Autodesk Inventor part; units mm, degrees
ref_plane "YZ Plane" through (0, 0, 0) normal (1, 0, 0) x (0, 1, 0)
ref_plane "XZ Plane" through (0, 0, 0) normal (0, 1, 0) x (-1, 0, 0)
ref_plane "XY Plane" through (0, 0, 0) normal (0, 0, 1) x (1, 0, 0)
sketch "Sketch1" plane through (0, 0, 0) normal (0, 0, 1) x (1, 0, 0)
  line L0 (0, 0) -> (30, 0)
  line L1 (30, 0) -> (30, 10)
  line L2 (30, 10) -> (0, 10)
  line L3 (0, 10) -> (0, 0)
  circle A0 centre (4, 5) radius 1.5
  circle A1 centre (26, 5) radius 1.5
  point P0 (0, 5)
  dimension "d0" = 30
  dimension "d1" = 10
  dimension "d22" = 3
  dimension "d23" = 3
  dimension "d24" = 4
  dimension "d25" = 4
extrude "Extrusion1" add sketch "Sketch1" along normal blind 5
sketch "Sketch2" plane through (0, 0, 5) normal (0, 0, 1) x (1, 0, 0)
  line L0 (30, 10) -> (0, 10)
  line L1 (0, 0) -> (30, 0)
  line L2 (7.5, 10) -> (22.5, 10)
  line L3 (22.5, 10) -> (22.5, 6)
  line L4 (22.5, 6) -> (7.5, 6)
  line L5 (7.5, 6) -> (7.5, 10)
  line L6 (7.5, 0) -> (22.5, 0)
  line L7 (22.5, 0) -> (22.5, 4)
  line L8 (22.5, 4) -> (7.5, 4)
  line L9 (7.5, 4) -> (7.5, 0)
  point P0 (15, 10)
  point P1 (15, 10)
  point P2 (15, 0)
  point P3 (15, 0)
  dimension "d14" = 15
  dimension "d15" = 15
  dimension "d31" = 2
  dimension "d32" = 4
  dimension "d33" = 4
extrude "Extrusion2" add sketch "Sketch2" along normal blind 7
fillet "Fillet1" radius 1 2 edges at (15, 6, 12) (15, 4, 12)
sketch "Sketch3" plane through (0, 0, 5) normal (0, 0, 1) x (1, 0, 0)
  circle A0 centre (4, 5) radius 1.5
  circle A1 centre (26, 5) radius 1.5
  circle A2 centre (4, 5) radius 3
  circle A3 centre (26, 5) radius 3
  point P0 (0, 0)
  dimension "d35" = 6
  dimension "d36" = 6
extrude "Extrusion3" cut sketch "Sketch3" against normal blind 3
equation "\"d15\" = d14"
equation "\"d32\" = d33"
properties part number "GT2 grip n roll"
Geometry check sheet. Reference: the model listing, model coordinates, mm. A direction names the side the tool comes from. Give positions to 0.01 mm unless a question says otherwise; leave off trailing zeros. Order: outer loops, then holes, each group sorted by start corner. A loop starts at its lowest first (then second) coordinate and runs counter-clockwise, first axis right, second up. Notation, with made-up numbers: (-22.5, 14) -> (24.5, 14) arc R9 cw to (24.5, 29) -> close; hole circle Ø3 at (-5.5, 63). An arc over 180 degrees is marked (long way). Write each question's results on one line, items separated by ' | '. Start each with the question number.
(1) Mould release check, pull along Y, two halves, no side actions. Record for faces 4 (the face through (0, 5, 2)), 5 (the face through (15, 6, 8)): pulls with the +Y half, pulls with the -Y half, needs draft (parallel to the pull), parting line crosses it, or undercut.
(2) Sectioned sample at C-C (x = 26). Enter the section's corners in (y, z), plus the area to 3 significant figures.
(3) Access from +Z, -Z, +X, -X, +Y, -Y to the whole of each face (thin tool, end or side, straight path). Record for faces 1 (the face through (14.895, 6.285, 11.699)), 2 (the face through (22.5, 2, 8)), 3 (the face through (1.6, 3.2, 3.5)).
(4) Sectioned sample at B-B (z = 6.5). Enter the section's corners in (x, y).
(5) Sectioned sample at D-D (x = 17.25). Enter the section's corners in (y, z).
(6) Scan lines: line 1 (Y direction, x = 26, z = 4.4); line 2 (X direction, y = 5.5, z = 2.5); line 3 (X direction, y = 6, z = 1). Record each from-to range of solid material in increasing order.
(7) Sectioned sample at A-A (y = 5). Enter the section's corners in (x, z).
(8) Gauge pin test, flat ends, axial feed: P1, Ø1.8, axis at x = 4, y = 4, coming from the +Z side; P2, Ø4.5, axis at y = 7.5, z = 8.5, coming from the -X side; P3, Ø5, axis at x = 27, y = 6, coming from the +Z side; P4, Ø2.5, axis at x = 4, y = 5, coming from the -Z side. Record the tip position at first contact, or that the pin passes through.
Answer below:
1) face 4: needs draft | face 5: undercut
2) outline: (0, 0) -> (3.5, 0) -> (3.5, 2) -> (2, 2) -> (2, 5) -> (0, 5) -> close; (6.5, 0) -> (10, 0) -> (10, 5) -> (8, 5) -> (8, 2) -> (6.5, 2) -> close | area: 26.0 mm2
3) face 1: +Z, +X, -X | face 2: +Z, +X, +Y, -Y | face 3: +Z
4) outline: (7.5, 0) -> (22.5, 0) -> (22.5, 4) -> (7.5, 4) -> close; (7.5, 6) -> (22.5, 6) -> (22.5, 10) -> (7.5, 10) -> close
5) outline: (0, 0) -> (10, 0) -> (10, 12) -> (7, 12) arc R1 ccw to (6, 11) -> (6, 5) -> (4, 5) -> (4, 11) arc R1 ccw to (3, 12) -> (0, 12) -> close
6) line 1: 0 to 2, 8 to 10 | line 2: 0 to 1.04, 6.96 to 23.04, 28.96 to 30 | line 3: 0 to 2.88, 5.12 to 24.88, 27.12 to 30
7) outline: (0, 0) -> (2.5, 0) -> (2.5, 2) -> (1, 2) -> (1, 5) -> (0, 5) -> close; (5.5, 0) -> (24.5, 0) -> (24.5, 2) -> (23, 2) -> (23, 5) -> (7, 5) -> (7, 2) -> (5.5, 2) -> close; (27.5, 0) -> (30, 0) -> (30, 5) -> (29, 5) -> (29, 2) -> (27.5, 2) -> close
8) P1: z = 2 | P2: x = 7.5 | P3: z = 5 | P4: through
